Geometry check sheet. Reference: drawing and pictorial views, mm from the part's lowest x, y, z. A direction names the side the tool comes from. Give positions to 0.01 mm unless a question says otherwise; leave off trailing zeros. Write each loop counter-clockwise with the first axis right and the second up, starting at its lowest first coordinate (ties: lowest second). Pieces come first, ordered by that corner, then holes.
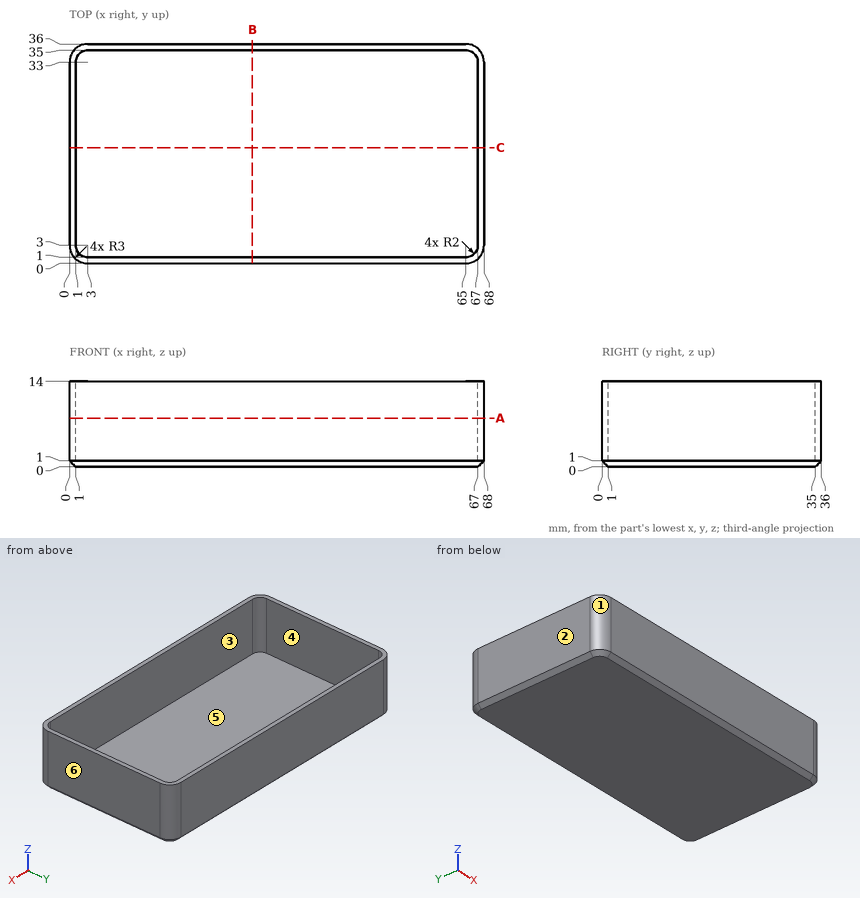
Item 1: Sectioned sample at C-C on y = 19. Record the cut outline in (x, z).
Answer key:
outline: (0, 1) - (1, 0) - (67, 0) - (68, 1) - (68, 14) - (67, 14) - (67, 1) - (1, 1) - (1, 14) - (0, 14) - close
Item 2: Sectioned sample at B-B on x = 30. Record the cut outline in (y, z), then the cut area to 3 significant figures.
Answer key:
outline: (0, 1) - (1, 0) - (35, 0) - (36, 1) - (36, 14) - (35, 14) - (35, 1) - (1, 1) - (1, 14) - (0, 14) - close
area: 61.0 mm2
Item 3: Scan lines: line 1 along X through (y, z) = (17, 10.5); line 2 along Y through (x, z) = (10, 13); line 3 along Z through (x, y) = (58, 27). Record each from-to range of solid material in increasing order.
Answer key:
line 1: x = 0 to 1, 67 to 68
line 2: y = 0 to 1, 35 to 36
line 3: z = 0 to 1
Item 4: Depth check by flat-ended pin: pin 1 (2 mm diameter, centred on x = 38, y = 13.5, fed in from +Z). Enter the tip coordinate at first touch or a pass-through.
Answer key:
pin 1: stops at z = 1
Item 5: Release check for a two-part mould opening along Y. For the marked faces 1, 2, 3 and 4 record: released by +Y, released by -Y, zero draft, split by the parting line, or undercut.
Answer key:
face 1: released by -Y
face 2: zero draft
face 3: undercut
face 4: undercut
Item 6: Sectioned sample at A-A on z = 8. Record the cut outline in (x, y), then the cut area to 3 significant figures.
Answer key:
outline: (0, 3) arc R3 ccw to (3, 0) - (65, 0) arc R3 ccw to (68, 3) - (68, 33) arc R3 ccw to (65, 36) - (3, 36) arc R3 ccw to (0, 33) - close; hole (1, 3) arc R2 ccw to (3, 1) - (65, 1) arc R2 ccw to (67, 3) - (67, 33) arc R2 ccw to (65, 35) - (3, 35) arc R2 ccw to (1, 33) - close
area: 200 mm2
Item 7: Set-up check for the marked faces 5 and 6: record each of +Z, -Z, +X, -X, +Y, -Y from which the full face is reachable in a straight line by a thin tool's end or side.
Answer key:
face 5: +Z
face 6: +Z, -Z, +X, +Y, -Y
